CAD build for the part. Positions are in the model's coordinates, mm. Face numbers are marked on the shaded views. A direction names the side the tool comes from. Give positions to 0.01 mm unless a question says otherwise; leave off trailing zeros. Loops run counter-clockwise (first coordinate to the right, second up) from the corner with the lowest first, then second, coordinate; pieces in that order, holes last.
```python
from build123d import *

# Parameters (mm, degrees)
SKETCH1_W           = 25.4
SKETCH1_H           = 7.62
BOSS_EXTRUDE1_DEPTH = 2.54
SKETCH3_W           = 2.54
SKETCH3_H           = 7.62
BOSS_EXTRUDE3_DEPTH = 25.4
FILLET1_RADIUS      = 3.81
FILLET1_LENGTH      = 2.54
SKETCH5_R           = 0.762
CUT_EXTRUDE1_DEPTH  = 25.4
FILLET2_RADIUS      = 3.81
FILLET2_LENGTH      = 2.54


with BuildPart() as part:
    # Sketch1 → Boss-Extrude1 (new body)
    with BuildSketch(Plane(origin=(0, 0, 0), x_dir=(1, 0, 0), z_dir=(0, 1, 0))):
        Rectangle(SKETCH1_W, SKETCH1_H)
    extrude(amount=BOSS_EXTRUDE1_DEPTH)

    # Sketch3 → Boss-Extrude3 (add)
    with BuildSketch(Plane(origin=(0, 2.54, 0), x_dir=(1, 0, 0), z_dir=(0, 1, 0))):
        with Locations((11.43, 0)):
            Rectangle(SKETCH3_W, SKETCH3_H)
    extrude(amount=BOSS_EXTRUDE3_DEPTH)

    # Fillet1: full round fillet: the end face becomes a half cylinder, R = half its width
    fillet1_face = Plane((-12.7, 1.27, 0), x_dir=(0, -1, 0), z_dir=(-1, 0, 0))  # on the end face: x along it, z out of the body
    fillet1_slab = fillet1_face.offset(-FILLET1_RADIUS / 2) * Box(FILLET1_LENGTH, 2 * FILLET1_RADIUS, FILLET1_RADIUS, mode=Mode.PRIVATE)  # the body's end, R deep
    fillet1_round = Plane((-8.89, 1.27, 0), x_dir=(-1, 0, 0), z_dir=(0, -1, 0)) * Cylinder(FILLET1_RADIUS, FILLET1_LENGTH, mode=Mode.PRIVATE)  # its axis R under the face
    add(fillet1_slab - fillet1_round, mode=Mode.SUBTRACT)

    # Sketch5 → Cut-Extrude1 (cut)
    with BuildSketch(Plane.ZY.offset(-10.16)):
        with Locations((0, 25.531689307)):
            Circle(SKETCH5_R)
    extrude(amount=-CUT_EXTRUDE1_DEPTH, mode=Mode.SUBTRACT)

    # Fillet2: full round fillet: the end face becomes a half cylinder, R = half its width
    fillet2_face = Plane((11.43, 27.94, 0), x_dir=(-1, 0, 0), z_dir=(0, 1, 0))  # on the end face: x along it, z out of the body
    fillet2_slab = fillet2_face.offset(-FILLET2_RADIUS / 2) * Box(FILLET2_LENGTH, 2 * FILLET2_RADIUS, FILLET2_RADIUS, mode=Mode.PRIVATE)  # the body's end, R deep
    fillet2_round = Plane((11.43, 24.13, 0), x_dir=(0, 1, 0), z_dir=(-1, 0, 0)) * Cylinder(FILLET2_RADIUS, FILLET2_LENGTH, mode=Mode.PRIVATE)  # its axis R under the face
    add(fillet2_slab - fillet2_round, mode=Mode.SUBTRACT)


solid = part.part
```
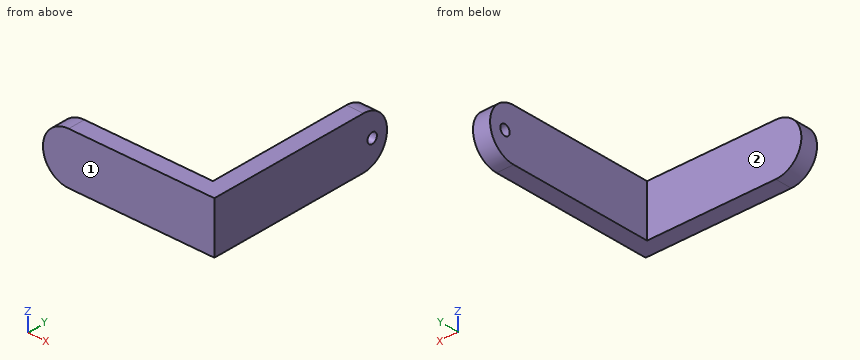
1. Saw through at A-A, the plane z = 0. List the corners of the cut face in (x, y), and give its area (3 significant figures).
Responses:
outline: (-12.7, 0) - (12.7, 0) - (12.7, 24.77) - (10.16, 24.77) - (10.16, 2.54) - (-12.7, 2.54) - close; (10.16, 26.29) - (12.7, 26.29) - (12.7, 27.94) - (10.16, 27.94) - close
area: 125 mm2
2. Probe line 1 along Y through (x, z) = (11.2, 0); line 2 along X through (y, z) = (23.5, 3); line 3 along Y through (x, z) = (8.5, 1.25). List the from-to ranges inside material, lowest first.
Responses:
line 1: y = 0 to 24.77, 26.29 to 27.94
line 2: x = 10.16 to 12.7
line 3: y = 0 to 2.54
3. Tool access for the marked faces 1 and 2: list every direction of +Z, -Z, +X, -X, +Y, -Y with a clear straight run to the whole face (end or side of a thin tool).
Responses:
face 1: +Z, -Z, +X, -X, -Y
face 2: +Z, -Z, -X, +Y
4. Saw through at D-D, the plane z = -1.75. List the corners of the cut face in (x, y).
Responses:
outline: (-12.27, 0) - (12.7, 0) - (12.7, 27.51) - (10.16, 27.51) - (10.16, 2.54) - (-12.27, 2.54) - close
5. Saw through at C-C, the plane x = 2.75. List the corners of the cut face in (y, z), and give its area (3 significant figures).
Responses:
outline: (0, -3.81) - (2.54, -3.81) - (2.54, 3.81) - (0, 3.81) - close
area: 19.4 mm2
6. Saw through at B-B, the plane y = 14.5. List the corners of the cut face in (x, z), and give its area (3 significant figures).
Responses:
outline: (10.16, -3.81) - (12.7, -3.81) - (12.7, 3.81) - (10.16, 3.81) - close
area: 19.4 mm2
7. Drop flat-ended pins along their axis: pin 1 (2 mm diameter, centred on x = -3.5, z = -1, fed in from -Y); pin 2 (2.5 mm diameter, centred on y = 14.5, z = -1, fed in from -X). Give the stop position or say it passes through.
Responses:
pin 1: stops at y = 0
pin 2: stops at x = 10.16
